Read the model definition and answer for the solid it produces. Units are mm, in the model's axes. A direction names the side the tool comes from. Give positions to 0.01 mm unless a question says otherwise; leave off trailing zeros. Write each loop counter-clockwise with the first axis right and the second up, starting at its lowest first coordinate (ties: lowest second). Pieces come first, ordered by that corner, then holes. Notation, with made-up numbers: (85.25, 86.25) - (100.25, 86.25) arc R21 ccw to (100.25, 109.25) - close; hole circle Ø8 at (40.25, 1.25). An arc over 180 degrees is marked (long way). Answer as CSV lines item,"result".
```python
from build123d import *

# Parameters (mm, degrees)
SKETCH1_W           = 28
SKETCH1_H           = 16
BOSS_EXTRUDE1_DEPTH = 18
SKETCH3_W           = 10
SKETCH3_H           = 10
BOSS_EXTRUDE2_DEPTH = 20
SKETCH4_W           = 12
SKETCH4_H           = 14
CUT_EXTRUDE1_DEPTH  = 25
SKETCH5_R           = 1.5
CUT_EXTRUDE2_DEPTH  = 25
SKETCH4_2_W         = 12
SKETCH4_2_H         = 14
CUT_EXTRUDE3_DEPTH  = 26


with BuildPart() as part:
    # Sketch1 → Boss-Extrude1 (new body)
    with BuildSketch(Plane(origin=(0, 0, 0), x_dir=(1, 0, 0), z_dir=(0, 1, 0))):
        with Locations((0.461538462, -2.646153846)):
            Rectangle(SKETCH1_W, SKETCH1_H)
    extrude(amount=BOSS_EXTRUDE1_DEPTH)

    # Sketch3 → Boss-Extrude2 (add)
    with BuildSketch(Plane.XY.offset(10.646153846)):
        with Locations((-1.538461538, 9)):
            Rectangle(SKETCH3_W, SKETCH3_H)
    extrude(amount=BOSS_EXTRUDE2_DEPTH)

    # Sketch4 → Cut-Extrude1 (cut)
    with BuildSketch(Plane(origin=(14.461538462, 0, 0), x_dir=(0, 0, -1), z_dir=(1, 0, 0))):
        with Locations((-2.646153846, 9)):
            Rectangle(SKETCH4_W, SKETCH4_H)
    extrude(amount=-CUT_EXTRUDE1_DEPTH, mode=Mode.SUBTRACT)

    # Sketch5 → Cut-Extrude2 (cut)
    with BuildSketch(Plane(origin=(0, 14, 0), x_dir=(1, 0, 0), z_dir=(0, 1, 0))):
        with Locations((-1.538461538, -20.646153846)):
            Circle(SKETCH5_R)
        with Locations((-1.538461538, -25.646153846)):
            Circle(SKETCH5_R)
    extrude(amount=-CUT_EXTRUDE2_DEPTH, mode=Mode.SUBTRACT)

    # Sketch4<2> → Cut-Extrude3 (cut)
    with BuildSketch(Plane(origin=(14.461538462, 0, 0), x_dir=(0, 0, -1), z_dir=(1, 0, 0))):
        with Locations((-2.646153846, 9)):
            Rectangle(SKETCH4_2_W, SKETCH4_2_H)
    extrude(amount=-CUT_EXTRUDE3_DEPTH, mode=Mode.SUBTRACT)


solid = part.part
```
(1) A cutting plane is placed at B-B (y = 3.5). Write down the section's boundary in (x, z).
Worked out:
outline,"(-13.54, -5.35) - (14.46, -5.35) - (14.46, -3.35) - (-11.54, -3.35) - (-11.54, 8.65) - (14.46, 8.65) - (14.46, 10.65) - (-13.54, 10.65) - close"
(2) Find the intervals of material crossed by L1, parallel to Y at x = 2.5, z = 7; L2, parallel to Z at x = -5.25, y = 4.75; L3, parallel to Z at x = 1.25, y = 15, in increasing order.
Worked out:
L1,"y = 0 to 2, 16 to 18"
L2,"z = -5.35 to -3.35, 8.65 to 30.65"
L3,"z = -5.35 to -3.35, 8.65 to 10.65"
(3) The mould has two halves that part along Y. Classify faces 6 (the flat face through (0, 9, -5.354)), 7 (the flat face through (0, 18, 3)), 8 (the flat face through (-11.538, 9, 3)): +Y half, -Y half, draft (parallel to the pull), parting line (faces both ways), or undercut.
Worked out:
face 6,"draft"
face 7,"+Y half"
face 8,"undercut"
(4) A cutting plane is placed at A-A (x = -3.75). Write down the section's boundary in (y, z), and give its area (3 significant figures).
Worked out:
outline,"(0, -5.35) - (18, -5.35) - (18, 10.65) - (14, 10.65) - (14, 30.65) - (4, 30.65) - (4, 10.65) - (0, 10.65) - close; hole (2, -3.35) - (16, -3.35) - (16, 8.65) - (2, 8.65) - close"
area,"320 mm^2"
(5) For faces 1 (the flat face through (3.462, 9, 21)), 2 (the flat face through (-2, 14, 18)), 3 (the flat face through (-2, 4, 18)), 4 (the flat face through (-6.538, 9, 21)), 5 (the flat face through (2, 9, -3.354)), determine the directions among +Z, -Z, +X, -X, +Y, -Y from which every point of the face is accessible in a straight line to the end or side of a thin tool.
Worked out:
face 1,"+Z, +X, +Y, -Y"
face 2,"+Z, +X, -X, +Y"
face 3,"+Z, +X, -X, -Y"
face 4,"+Z, -X, +Y, -Y"
face 5,"+X"
(6) A cutting plane is placed at C-C (z = 5). Write down the section's boundary in (x, y), and give its area (3 significant figures).
Worked out:
outline,"(-13.54, 0) - (14.46, 0) - (14.46, 2) - (-11.54, 2) - (-11.54, 16) - (14.46, 16) - (14.46, 18) - (-13.54, 18) - close"
area,"140 mm^2"
(7) A cutting plane is placed at D-D (x = -7.5). Write down the section's boundary in (y, z), and give its area (3 significant figures).
Worked out:
outline,"(0, -5.35) - (18, -5.35) - (18, 10.65) - (0, 10.65) - close; hole (2, -3.35) - (16, -3.35) - (16, 8.65) - (2, 8.65) - close"
area,"120 mm^2"
(8) Each of these flat-tipped pins is pushed along its axis until it touches: P1, Ø3, axis at y = 11, z = 23, coming from the +X side; P2, Ø10, axis at x = -0.5, z = 20, coming from the +Y side; P3, Ø5, axis at y = 10.5, z = 24, coming from the -X side. Where does it stop, or does it pass through?
Worked out:
P1,"stops at x = 3.46"
P2,"stops at y = 14"
P3,"stops at x = -6.54"
